Read the model definition and answer for the solid it produces. Units are mm, in the model's axes. A direction names the side the tool comes from. Coordinates: 2 decimals unless noted, no trailing zeros. Write each loop counter-clockwise with the first axis right and the second up, starting at its lowest first coordinate (ties: lowest second). Pieces come first, ordered by that corner, then holes.
Item 1: Section B-B (y = 6.75) is taken. Give the vertices of the cut face in (x, z), then the cut area to 3 significant figures.
Item 2: A tool of negligible diameter and unlimited length cuts with its end or side. For faces 1 (the face through (0, 11, 1.12)), 2 (the face through (0, 7, -3.8)), 3 (the face through (3.276, 7.478, 1.927)), 4 (the face through (-3.276, 7.478, -1.927)), from which of +Z, -Z, +X, -X, +Y, -Y can it reach the whole face along a straight path? Write none if from no direction.
Item 3: Each of these flat-tipped pins is pushed along its axis until it touches: P1, Ø0.5, axis at x = 0.5, z = -0.5, coming from the -Y side; P2, Ø1.3, axis at x = -0.5, z = -1, coming from the +Y side; P3, Ø1, axis at x = -0.5, y = 8, coming from the -Z side. Where does it stop, or does it pass through?
Item 4: Determine the mould class of faces 5 (the face through (0, 3, -5)), 6 (the face through (0.3, 7, 0)), 7 (the face through (4.35, 12.009, 2.465)), 8 (the face through (0.763, 2.982, 0.24)) for opening direction Z: released by +Z, released by -Z, zero draft, split by the parting line, or undercut.
Item 5: Straight lines are drawn through the part: probe 1 along Y at (x, z) = (-2.5, -4); probe 2 along Z at (x, y) = (0, 5); probe 3 along X at (y, z) = (3.5, 1.75). For each, find the intervals that lie inside material, in ascending order.
Item 6: Section D-D (z = 2) is taken. Give the vertices of the cut face in (x, y), then the cut area to 3 significant figures.
Item 7: Section A-A (z = 4.25) is taken. Give the vertices of the cut face in (x, y), then the cut area to 3 significant figures.
Item 8: Section C-C (x = 4.75) is taken. Give the vertices of the cut face in (y, z), then the cut area to 3 significant figures.
Autodesk Inventor part; units mm, degrees
ref_plane "Plano de trabajo1" through (0, 7.5, 0) normal (0, 1, 0) x (1, 0, 0)
ref_plane "YZ Plane" through (0, 0, 0) normal (1, 0, 0) x (0, 1, 0)
ref_plane "XZ Plane" through (0, 0, 0) normal (0, 1, 0) x (-1, 0, 0)
sketch "Boceto1" plane through (0, 0, 0) normal (0, 1, 0) x (-1, 0, 0)
  line L0 (5.7735, 0) -> (2.8868, -5)
  line L1 (2.8868, -5) -> (-2.8868, -5)
  line L2 (-2.8868, -5) -> (-5.7735, 0)
  line L3 (-5.7735, 0) -> (-2.8868, 5)
  line L4 (-2.8868, 5) -> (2.8868, 5)
  line L5 (2.8868, 5) -> (5.7735, 0)
  circle A0 centre (0, 0) radius 5
  dimension "d0" = 10
extrude "Extrusión1" add sketch "Boceto1" along normal blind 15
sketch "Boceto2" plane through (0, 15, 0) normal (0, 1, 0) x (1, 0, 0)
  circle A0 centre (0, 0) radius 1.575
  line L0 (-1.1074, -1.12) -> (1.1074, -1.12)
  dimension "d3" = 3.15
  dimension "d6" = 1.12
extrude "Extrusión2" cut sketch "Boceto2" against normal blind 7 contours A0 L0 picked at (0.4242, -0.1216)
sketch "Boceto3" plane through (0, 0, 0) normal (0, -1, 0) x (1, 0, 0)
  circle A0 centre (0, 0) radius 0.8
  dimension "d7" = 1.6
extrude "Extrusión3" cut sketch "Boceto3" against normal blind 7
sketch "Boceto4" plane through (0, 7, 0) normal (0, -1, 0) x (1, 0, 0)
  circle A0 centre (0, 0) radius 0.8
  line L0 (0.1389, -0.7878) -> (-0.1389, 0.7878)
  circle A1 centre (0, 0) radius 0.8
  line L1 (0.8, 0) -> (-0.8, 0)
  line L2 (-0.0393, 0.799) -> (0.2363, -0.7643)
  line L3 (0.0894, -0.795) -> (-0.1879, 0.7776)
  point P0 (0.0894, -0.795)
  point P1 (-0.1879, 0.7776)
  dimension "d16" = 80
  dimension "d17" = 0.1
  dimension "d18" = 0.05
extrude "Extrusión4" add sketch "Boceto4" along normal blind 2 contours L0 L1 L3 A0 | A0 L3 L1 L0 | L3 L1 A0 | A0 L1 L3
ref_plane "Plano de trabajo1" through (0, 7.5, 0) normal (0, 1, 0) x (1, 0, 0)
sketch "Boceto5" plane through (0, 7.5, 0) normal (0, 1, 0) x (1, 0, 0)
  circle A0 centre (0, 0) radius 0.8
  line L0 (5.7735, 0) -> (2.8868, 5)
  line L1 (2.8868, -5) -> (5.7735, 0)
  line L2 (-2.8868, -5) -> (2.8868, -5)
  line L3 (-5.7735, 0) -> (-2.8868, -5)
  line L4 (-2.8868, 5) -> (-5.7735, 0)
  line L5 (2.8868, 5) -> (-2.8868, 5)
  line L6 (-4.3879, 0) -> (-2.1939, -3.8)
  line L7 (-2.1939, -3.8) -> (2.1939, -3.8)
  line L8 (2.1939, -3.8) -> (4.3879, 0)
  line L9 (4.3879, 0) -> (2.1939, 3.8)
  line L10 (2.1939, 3.8) -> (-2.1939, 3.8)
  line L11 (-2.1939, 3.8) -> (-4.3879, 0)
  arc A1 (-0.1389, -0.7878) -> (0.1389, 0.7878) centre (0, 0) ccw
  circle A2 centre (0, 0) radius 6.7948
  point P0 (-0.1792, -0.7283)
  point P1 (0.0807, 0.7456)
  dimension "d13" = 1.2
extrude "Extrusión5" cut sketch "Boceto5" along normal mid plane 3.2 contours L1 L2 L3 L4 L5 L0
fillet "Empalme2" radius 0.5 3 edges at (-0.8, 0, 0) (0, 15, -1.575) (0, 15, 1.12)
fillet "Empalme3" radius 0.5 1 edges at (0, 5, 0)
properties part number "Couple"
Established:
1. outline: (-4.39, 0) - (-2.19, -3.8) - (2.19, -3.8) - (4.39, 0) - (2.19, 3.8) - (-2.19, 3.8) - close; hole (-0.14, 0.79) - (0.14, -0.79) arc R0.8 ccw to start
1. area: 49.0 mm2
2. face 1: +Y
2. face 2: -Z, +X, -X
2. face 3: +Z, +X
2. face 4: -Z, -X
3. P1: stops at y = 0.14
3. P2: stops at y = 14.89
3. P3: stops at z = -3.8
4. face 5: released by -Z
4. face 6: undercut
4. face 7: released by +Z
4. face 8: undercut
5. probe 1: y = 0 to 5.9, 9.1 to 15
5. probe 2: z = -5 to -0.8, 0.8 to 5
5. probe 3: x = -4.76 to 4.76
6. outline: (-4.62, 0) - (4.62, 0) - (4.62, 5.9) - (3.23, 5.9) - (3.23, 9.1) - (4.62, 9.1) - (4.62, 15) - (-4.62, 15) - (-4.62, 9.1) - (-3.23, 9.1) - (-3.23, 5.9) - (-4.62, 5.9) - close
6. area: 130 mm2
7. outline: (-3.32, 0) - (3.32, 0) - (3.32, 5.9) - (-3.32, 5.9) - close; (-3.32, 9.1) - (3.32, 9.1) - (3.32, 15) - (-3.32, 15) - close
7. area: 78.3 mm2
8. outline: (0, -1.77) - (5.9, -1.77) - (5.9, 1.77) - (0, 1.77) - close; (9.1, -1.77) - (15, -1.77) - (15, 1.77) - (9.1, 1.77) - close
8. area: 41.8 mm2
